Check sheet for the modelled part. Datum: model origin and axes. Units: mm. A direction names the side the tool comes from. Give positions to 0.01 mm unless a question says otherwise; leave off trailing zeros. Order: outer loops, then holes, each group sorted by start corner. A loop starts at its lowest first (then second) coordinate and runs counter-clockwise, first axis right, second up.
from build123d import *

# Parameters (mm, degrees)
SKETCH1_R                = 1.55
SKETCH1_R_2              = 7
SKETCH1_R_3              = 2.5
BOSS_EXTRUDE1_DEPTH      = 20
BOSS_EXTRUDE2_REACH      = 53.813
BOSS_EXTRUDE2_END_RADIUS = 18.9
BOSS_EXTRUDE3_REACH      = 55.526
BOSS_EXTRUDE3_END_RADIUS = 18.9
SKETCH3_W                = 6
SKETCH3_H                = 20
SKETCH5_R                = 1.675
CUT_EXTRUDE3_DEPTH       = 22.5
CUT_EXTRUDE4_DEPTH       = 11
CUT_EXTRUDE5_DEPTH       = 5.25
SKETCH8_R                = 1.06
CUT_EXTRUDE6_DEPTH       = 54.525694884
SKETCH9_R                = 3
CUT_EXTRUDE7_DEPTH       = 10
SKETCH11_R               = 11.2
CUT_EXTRUDE9_DEPTH       = 2.35
CUT_EXTRUDE8_DEPTH       = 6
SKETCH15_W               = 3
SKETCH15_H               = 68
BOSS_EXTRUDE5_DEPTH      = 20
FILLET2_R                = 3
CUT_EXTRUDE11_REACH      = 61.674
SKETCH16_R               = 1.75


with BuildPart() as part:
    # Sketch1 → Boss-Extrude1 (new body)
    with BuildSketch(Plane(origin=(0, 0, 0), x_dir=(1, 0, 0), z_dir=(0, 1, 0))):
        with BuildLine():
            Line((10.349494937, -15.814485593), (10.349494937, 8.416255239))
            ThreePointArc((10.349494937, 8.416255239), (10.822804202, 11.144484896), (8.349494937, 9.899494937))
            Line((8.349494937, 9.899494937), (8.349494937, -16.955705067))
            ThreePointArc((8.349494937, -16.955705067), (-17.76919177, 6.439396233), (17.273666667, 7.670100383))
            ThreePointArc((17.273666667, 7.670100383), (23, 0), (17.273666667, -7.670100383))
            ThreePointArc((17.273666667, -7.670100383), (14.399392933, -12.242037541), (10.349494937, -15.814485593))
        make_face()
        with Locations(Location((-9.899494937, 9.899494937, 0), (0, 0, 270))):
            Circle(SKETCH1_R, mode=Mode.SUBTRACT)
        with Locations(Location((-9.899494937, -9.899494937, 0), (0, 0, 270))):
            Circle(SKETCH1_R, mode=Mode.SUBTRACT)
        with Locations(Location((0, 0, 0), (0, 0, 270))):
            Circle(SKETCH1_R_2, mode=Mode.SUBTRACT)
        with Locations(Location((15, 0, 0), (0, 0, 270))):
            Circle(SKETCH1_R_3, mode=Mode.SUBTRACT)
    extrude(amount=BOSS_EXTRUDE1_DEPTH)

    # Boss-Extrude2: up to this cylinder (the profile starts outside it)
    boss_extrude2_end = Plane(origin=(0, 6.495191, 0), z_dir=(0, -1, 0)) * Cylinder(BOSS_EXTRUDE2_END_RADIUS, 146.426, mode=Mode.PRIVATE)
    # Sketch2 → Boss-Extrude2 (add, up to the surface)
    with BuildSketch(Plane.XY.offset(-23), mode=Mode.PRIVATE) as boss_extrude2_sk1:
        Polygon((14.1, 6.495190528), (10.35, 0), (2.85, 0), (-0.9, 6.495190528), (2.85, 12.990381057), (10.35, 12.990381057), align=None)
    boss_extrude2_tool1 = extrude(boss_extrude2_sk1.sketch, amount=BOSS_EXTRUDE2_REACH, mode=Mode.PRIVATE) - boss_extrude2_end
    add(boss_extrude2_tool1.solids().sort_by_distance((6.6, 6.495191, -23))[0])

    # Boss-Extrude3: up to this cylinder (the profile starts outside it)
    boss_extrude3_end = Plane(origin=(0, 9.928375, 0), z_dir=(0, -1, 0)) * Cylinder(BOSS_EXTRUDE3_END_RADIUS, 149.99525, mode=Mode.PRIVATE)
    # Sketch3 → Boss-Extrude3 (add, up to the surface)
    with BuildSketch(Plane.XY.offset(21), mode=Mode.PRIVATE) as boss_extrude3_sk1:
        with BuildLine():
            Line((8.349494937, 20), (3.349494937, 20))
            Line((3.349494937, 20), (3.349494937, 8.936698586))
            ThreePointArc((3.349494937, 8.936698586), (2.099494937, 6.5), (3.349494937, 4.063301414))
            Line((3.349494937, 4.063301414), (3.349494937, 0))
            Line((3.349494937, 0), (8.349494937, 0))
            Line((8.349494937, 0), (8.349494937, 20))
        make_face()
    boss_extrude3_tool1 = extrude(boss_extrude3_sk1.sketch, amount=-BOSS_EXTRUDE3_REACH, mode=Mode.PRIVATE) - boss_extrude3_end
    add(boss_extrude3_tool1.solids().sort_by_distance((5.726294, 9.85675, 21))[0])
    # Sketch3 → Boss-Extrude3 (add, up to the surface)
    with BuildSketch(Plane.XY.offset(21), mode=Mode.PRIVATE) as boss_extrude3_sk2:
        with Locations((13.349494937, 10)):
            Rectangle(SKETCH3_W, SKETCH3_H)
    boss_extrude3_tool2 = extrude(boss_extrude3_sk2.sketch, amount=-BOSS_EXTRUDE3_REACH, mode=Mode.PRIVATE) - boss_extrude3_end
    add(boss_extrude3_tool2.solids().sort_by_distance((13.349495, 10, 21))[0])

    # Sketch5 → Cut-Extrude3 (cut)
    with BuildSketch(Plane(origin=(16.349494937, 0, 0), x_dir=(0, 0, -1), z_dir=(1, 0, 0))):
        with Locations(Location((-17, 12, 0), (0, 0, 90))):
            Circle(SKETCH5_R)
    extrude(amount=-CUT_EXTRUDE3_DEPTH, mode=Mode.SUBTRACT)

    # Sketch6 → Cut-Extrude4 (cut)
    with BuildSketch(Plane(origin=(-6.150505063, 0, 0), x_dir=(0, 0, -1), z_dir=(1, 0, 0))):
        Polygon((-20.35, 12), (-18.675, 9.098814897), (-15.325, 9.098814897), (-13.65, 12), (-15.325, 14.901185103), (-18.675, 14.901185103), align=None)
    extrude(amount=CUT_EXTRUDE4_DEPTH, mode=Mode.SUBTRACT)

    # Sketch7 → Cut-Extrude5 (cut)
    with BuildSketch(Plane(origin=(0, 4.25, 0), x_dir=(1, 0, 0), z_dir=(0, 1, 0))):
        with BuildLine():
            Line((6.29798001, 4), (5.744562647, 4))
            Line((5.744562647, 4), (5.744562647, -4))
            Line((5.744562647, -4), (6.29798001, -4))
            ThreePointArc((6.29798001, -4), (24.577324882, 0), (6.29798001, 4))
        make_face()
    extrude(amount=CUT_EXTRUDE5_DEPTH, mode=Mode.SUBTRACT)

    # Sketch8 → Cut-Extrude6 (cut, through all)
    with BuildSketch(Plane(origin=(0, 0, -23), x_dir=(-1, 0, 0), z_dir=(0, 0, -1))):
        with Locations((-6.6, 6.495190528)):
            Circle(SKETCH8_R)
    extrude(amount=-CUT_EXTRUDE6_DEPTH, mode=Mode.SUBTRACT)

    # Sketch9 → Cut-Extrude7 (cut)
    with BuildSketch(Plane(origin=(0, 0, -23), x_dir=(-1, 0, 0), z_dir=(0, 0, -1))):
        with Locations((-6.6, 6.495190528)):
            Circle(SKETCH9_R)
    extrude(amount=-CUT_EXTRUDE7_DEPTH, mode=Mode.SUBTRACT)

    # Sketch11 → Cut-Extrude9 (cut)
    with BuildSketch(Plane(origin=(0, 20, 0), x_dir=(1, 0, 0), z_dir=(0, 1, 0))):
        Circle(SKETCH11_R)
    extrude(amount=-CUT_EXTRUDE9_DEPTH, mode=Mode.SUBTRACT)

    # Sketch10 → Cut-Extrude8 (cut)
    with BuildSketch(Plane(origin=(0, 20, 0), x_dir=(1, 0, 0), z_dir=(0, 1, 0))):
        Polygon((15, 4.7), (10.929680602, 2.35), (10.349494937, 2.35), (10.349494937, -2.35), (10.929680602, -2.35), (15, -4.7), (19.070319398, -2.35), (19.070319398, 2.35), align=None)
    extrude(amount=-CUT_EXTRUDE8_DEPTH, mode=Mode.SUBTRACT)

    # Cut-Revolve1: read off the stored shape, not the designer's step
    # Cut-Revolve1: loft between two sections, ruled curve by curve
    cut_revolve1_from = [
        Edge.make_three_point_arc((7.653578644, 6.608263478, -9.001288479), (6.491231459, 7.554083708, -9.001288479), (5.545411229, 6.391736522, -9.001288479)),
        Edge.make_three_point_arc((5.545411229, 6.391736522, -9.001288479), (6.707758415, 5.445916292, -9.001288479), (7.653578644, 6.608263478, -9.001288479)),
    ]
    cut_revolve1_to = [
        Edge.make_three_point_arc((9.086412031, 6.755427811, -4), (6.344067126, 8.986917094, -4), (4.112577842, 6.244572189, -4)),
        Edge.make_three_point_arc((4.112577842, 6.244572189, -4), (6.854922748, 4.013082906, -4), (9.086412031, 6.755427811, -4)),
    ]
    cut_revolve1 = Solid(Shell([*[Face.make_surface_from_curves(cut_revolve1_from[k], cut_revolve1_to[k]) for k in range(2)], Face(Wire(cut_revolve1_from)), Face(Wire(cut_revolve1_to))]))
    add(cut_revolve1, mode=Mode.SUBTRACT)

    # Sketch15 → Boss-Extrude5 (add)
    with BuildSketch(Plane(origin=(0, 0, 0), x_dir=(1, 0, 0), z_dir=(0, 1, 0))):
        with Locations((-19.5, 1)):
            Rectangle(SKETCH15_W, SKETCH15_H)
    extrude(amount=BOSS_EXTRUDE5_DEPTH)

    # Fillet2
    fillet2_edges = [part.edges().sort_by_distance(p)[0] for p in [
        (-18, 10, -5.762811814),
        (-18, 10, 5.762811814),
    ]]
    fillet(fillet2_edges, radius=FILLET2_R)

    # Sketch16 → Cut-Extrude11 (cut, up to next)
    with BuildSketch(Plane.ZY.offset(21), mode=Mode.PRIVATE) as cut_extrude11_sk1:
        with Locations((-27, 10)):
            Circle(SKETCH16_R)
    cut_extrude11_tool1 = extrude(cut_extrude11_sk1.sketch, amount=-CUT_EXTRUDE11_REACH, mode=Mode.PRIVATE) & part.part
    # Sketch16 → Cut-Extrude11 (cut, up to next)
    with BuildSketch(Plane.ZY.offset(21), mode=Mode.PRIVATE) as cut_extrude11_sk2:
        with Locations((27, 10)):
            Circle(SKETCH16_R)
    cut_extrude11_tool2 = extrude(cut_extrude11_sk2.sketch, amount=-CUT_EXTRUDE11_REACH, mode=Mode.PRIVATE) & part.part
    add(cut_extrude11_tool1.solids().sort_by_distance((-21, 10, -27))[0], mode=Mode.SUBTRACT)
    add(cut_extrude11_tool2.solids().sort_by_distance((-21, 10, 27))[0], mode=Mode.SUBTRACT)


solid = part.part
1) Section check A-A, the plane z = -27. Record the cut outline in (x, y).
Recorded:
outline: (-21, 0) - (-18, 0) - (-18, 8.25) - (-21, 8.25) - close; (-21, 11.75) - (-18, 11.75) - (-18, 20) - (-21, 20) - close
2) Material ranges on L1, parallel to X at y = 10, z = 18; L2, parallel to X at y = 19, z = 12; L3, parallel to X at y = 8, z = -15, recorded low to high.
Recorded:
L1: x = -21 to -18, 4.85 to 8.35, 10.35 to 16.35
L2: x = -21 to 8.35, 10.35 to 16.35
L3: x = -21 to -17.84, -11.5 to 4, 9.2 to 13.23
3) Section check D-D, the plane z = 17. Record the cut outline in (x, y) (1 decimal), then the cut area to 3 significant figures.
Recorded:
outline: (-21, 0) - (-18, 0) - (-18, 20) - (-21, 20) - close; (-8.3, 0) - (8.3, 0) - (8.3, 10.3) - (4.8, 10.3) - (4.8, 9.1) - (-6.2, 9.1) - (-6.2, 14.9) - (4.8, 14.9) - (4.8, 13.7) - (8.3, 13.7) - (8.3, 20) - (-8.3, 20) - close; (10.3, 0) - (16.3, 0) - (16.3, 10.3) - (10.3, 10.3) - close; (10.3, 13.7) - (16.3, 13.7) - (16.3, 20) - (10.3, 20) - close; hole circle Ø2.1 at (6.6, 6.5)
area: 413 mm2
4) Draft check along Z on faces 1 (the face through (7.41, 7.42, 5.84)), 2 (the face through (23, 2, 0)), 3 (the face through (16.84, 14.68, 8.58)). Enter one of: +Z half, -Z half, draft (parallel to the pull), parting line (faces both ways), or undercut.
Recorded:
face 1: undercut
face 2: parting line
face 3: +Z half
5) Section check C-C, the plane x = 0. Record the cut outline in (y, z) (3 decimals).
Recorded:
outline: (0, -18.9) - (4.936, -18.9) - (4.936, -23) - (8.054, -23) - (8.054, -18.9) - (20, -18.9) - (20, -11.2) - (17.65, -11.2) - (17.65, -7) - (0, -7) - close; (0, 7) - (17.65, 7) - (17.65, 11.2) - (20, 11.2) - (20, 18.9) - (14.511, 18.9) - (14.901, 18.675) - (14.901, 15.325) - (12, 13.65) - (9.099, 15.325) - (9.099, 18.675) - (9.489, 18.9) - (0, 18.9) - close
6) Depth check by flat-ended pin: pin 1 Ø2 at (y, z) = (3.5, -23.5) entering from +X; pin 2 Ø0.5 at (x, y) = (10.5, 15) entering from +Z; pin 3 Ø8 at (x, y) = (-3, 17.5) entering from -Z. Enter the tip coordinate at first touch or a pass-through.
Recorded:
pin 1: stops at x = 12.87
pin 2: stops at z = 21
pin 3: stops at z = -18.9
7) Section check B-B, the plane z = 0. State how many separate pieces and enclosed holes the cut face has, then the cut area to 3 significant figures.
Recorded:
separate pieces: 7
enclosed holes: 0
area: 377 mm2
8) Set-up check for faces 4 (the face through (10.696, 18.841, -3.321)), 5 (the face through (12.2, 9.79, -19.02)), 6 (the face through (2.1, 6.5, 19.8)), 7 (the face through (3, 7, -23)): record each of +Z, -Z, +X, -X, +Y, -Y from which the full face is reachable in a straight line by a thin tool's end or side.
Recorded:
face 4: +Y
face 5: -Z, +X, +Y
face 6: +Z
face 7: -Z, +X, +Y, -Y
